Autodesk Fusion 360 part; units mm, degrees
sketch "Sketch1" plane through (0, 0, 0) normal (0, 0, 1) x (1, 0, 0)
  line L0 (12.5, -35) -> (-12.5, -35)
  line L1 (-12.5, -35) -> (-12.5, 35)
  line L2 (-12.5, 35) -> (12.5, 35)
  line L3 (12.5, 35) -> (12.5, -35)
  dimension "d1" = 70
  dimension "d2" = 25
  dimension "d3" = 12.5
  dimension "d4" = 35
extrude "Extrude1" add sketch "Sketch1" along normal blind 9
sketch "Sketch2" plane through (0, 0, 9) normal (0, 0, 1) x (-1, 0, 0)
  line L0 (-12.5, -35) -> (12.5, -35)
  line L1 (12.5, -35) -> (12.5, 35)
  line L2 (12.5, 35) -> (-12.5, 35)
  line L3 (-12.5, 35) -> (-12.5, -35)
  circle A0 centre (0, 0) radius 7.5
  line L4 (0, 0) -> (0, -29) construction
  line L5 (0, -29) -> (6.25, -29)
  circle A1 centre (6.25, -29) radius 2.5
  circle A2 centre (-6.25, -29) radius 2.5
  circle A3 centre (6.25, 29) radius 2.5
  circle A4 centre (-6.25, 29) radius 2.5
  dimension "d7" = 15
  dimension "d8" = 29
  dimension "d9" = 6.25
  dimension "d10" = 5
  dimension "d11" = 29
  dimension "d12" = 12.5
  dimension "d13" = 29
  dimension "d14" = 58
  dimension "d15" = 5
  dimension "d16" = 5
hole "Hole1" at (0, 0, 9) direction (0, 0, -1) diameter 15 depth 3 tip angle 118
hole "Hole2" at (-6.25, -29, 9) at (6.25, -29, 9) at (6.25, 29, 9) at (-6.25, 29, 9) direction (0, 0, -1) diameter 5 depth 7 tip angle 118
sketch "Sketch3" plane through (0, 0, 0) normal (0, 0, -1) x (1, 0, 0)
  line L0 (-12.5, -35) -> (12.5, -35)
  line L1 (12.5, -35) -> (12.5, 35)
  line L2 (12.5, 35) -> (-12.5, 35)
  line L3 (-12.5, 35) -> (-12.5, -35)
  circle A0 centre (0, 0) radius 9.5
  dimension "d23" = 19
hole "Hole3" at (0, 0, 0) direction (0, 0, 1) diameter 19 depth 6 tip angle 118
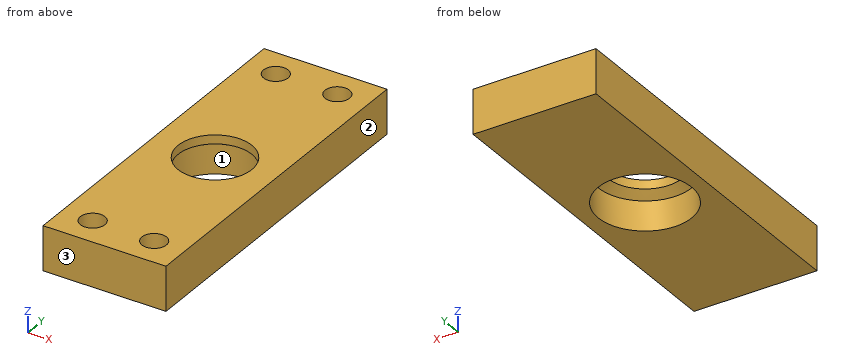
Design review of the part built by this model. Coordinates are the model's own, in mm. Face numbers are marked on the shaded views. Coordinates: 2 decimals unless noted, no trailing zeros. Write each loop counter-clockwise with the first axis right and the second up, starting at its lowest first coordinate (ties: lowest second). Pieces come first, ordered by that corner, then holes. Notation, with made-up numbers: (-7, -6.75) - (13, -6.75) arc R27 ccw to (13, 18.25) - close; hole circle Ø3 at (-0.5, 84). An arc over 180 degrees is marked (long way). Use one line per item in the form item = value.
Q1. For probe 1 along X at (y, z) = (-29, 7); probe 2 along X at (y, z) = (0, 4.05); probe 3 along Y at (x, z) = (7.25, 4.25), list the stretches that pass through material, from the lowest coordinate up.
Taken from the geometry:
probe_1 = -12.5 to -8.75, -3.75 to 3.75, 8.75 to 12.5
probe_2 = -12.5 to -9.5, 9.5 to 12.5
probe_3 = -35 to -31.29, -26.71 to -6.14, 6.14 to 26.71, 31.29 to 35
Q2. Consider section A-A (y = 0). Write out the cut boundary in (x, z), plus the area to 3 significant figures.
Taken from the geometry:
outline = (-12.5, 0) - (-9.5, 0) - (-9.5, 6) - (-7.5, 7.2) - (-7.5, 9) - (-12.5, 9) - close; (7.5, 7.2) - (9.5, 6) - (9.5, 0) - (12.5, 0) - (12.5, 9) - (7.5, 9) - close
area = 63.6 mm^2
Q3. Insertion check: pin 1 Ø4.5 at (x, y) = (-6.25, 29) entering from +Z. The pin has a flat end and moves straight along its axis. Give the tip position at first contact, or say it passes through.
Taken from the geometry:
pin_1 = 1.85
Q4. Consider section C-C (z = 3.75). Write out the cut boundary in (x, y), plus the area to 3 significant figures.
Taken from the geometry:
outline = (-12.5, -35) - (12.5, -35) - (12.5, 35) - (-12.5, 35) - close; hole circle Ø19 at (0, 0); hole circle Ø5 at (-6.25, -29); hole circle Ø5 at (-6.25, 29); hole circle Ø5 at (6.25, -29); hole circle Ø5 at (6.25, 29)
area = 1,390 mm^2
Q5. Consider section B-B (x = 0). Write out the cut boundary in (y, z).
Taken from the geometry:
outline = (-35, 0) - (-9.5, 0) - (-9.5, 6) - (-7.5, 7.2) - (-7.5, 9) - (-35, 9) - close; (7.5, 7.2) - (9.5, 6) - (9.5, 0) - (35, 0) - (35, 9) - (7.5, 9) - close
Q6. The part is to be moulded in two halves that separate along X. For the marked faces 1, 2 and 3, say which applies: +X half, -X half, draft (parallel to the pull), parting line (faces both ways), or undercut.
Taken from the geometry:
face_1 = undercut
face_2 = +X half
face_3 = draft
